from build123d import *

# Parameters (mm, degrees)
SKETCH_1_W          = 1.925
SKETCH_1_H          = 1.2
CUT_EXTRUDE_1_DEPTH = 1
SKETCH_3_W          = 0.8975
SKETCH_3_H          = 0.13363029
EXTRUDE_1_DEPTH     = 0.45
SKETCH_4_W          = 0.13363029
SKETCH_4_H          = 0.8975
EXTRUDE_2_DEPTH     = 0.45
SKETCH_5_W          = 0.8975
SKETCH_5_H          = 0.13363029
EXTRUDE_3_DEPTH     = 0.45
SKETCH_6_W          = 0.13363029
SKETCH_6_H          = 0.8975
EXTRUDE_4_DEPTH     = 0.45
SKETCH_7_R          = 1
EXTRUDE_5_DEPTH     = 6
DRAFT_1_ANGLE       = 30.706601503
DRAFT_2_ANGLE       = 30.706601503
DRAFT_3_ANGLE       = 30.706601503
DRAFT_4_ANGLE       = 30.706601503
FILLET_1_R          = 0.031496063
FILLET_2_R          = 0.45


with BuildPart() as part:
    # 草图1 → 旋转1 (revolve)
    with BuildSketch(Plane.XZ, mode=Mode.PRIVATE) as revolve_1_sk:
        with Locations((0.9625, 0.6)):
            Rectangle(SKETCH_1_W, SKETCH_1_H)
    revolve(revolve_1_sk.sketch.rotate(Axis((0, 0, 1.2), (0, 0, -1)), 270), axis=Axis((0, 0, 1.2), (0, 0, -1)))

    # 草图2 → 切除-拉伸1 (cut)
    with BuildSketch(Plane.XY.offset(1.2)):
        Polygon((0.225, 1.3475), (-0.225, 1.3475), (-0.225, 0.225), (-1.3475, 0.225), (-1.3475, -0.225), (-0.225, -0.225), (-0.225, -1.3475), (0.225, -1.3475), (0.225, -0.225), (1.3475, -0.225), (1.3475, 0.225), (0.225, 0.225), align=None)
    extrude(amount=-CUT_EXTRUDE_1_DEPTH, mode=Mode.SUBTRACT)

    # 草图3 → 凸台-拉伸1 (add)
    with BuildSketch(Plane.XZ.offset(-0.225)):
        with Locations((-0.89875, 0.266815145)):
            Rectangle(SKETCH_3_W, SKETCH_3_H)
    extrude(amount=EXTRUDE_1_DEPTH)

    # 草图4 → 凸台-拉伸2 (add)
    with BuildSketch(Plane(origin=(-0.225, 0, 0), x_dir=(0, 0, -1), z_dir=(1, 0, 0))):
        with Locations((-0.266815145, 0.89875)):
            Rectangle(SKETCH_4_W, SKETCH_4_H)
    extrude(amount=EXTRUDE_2_DEPTH)

    # 草图5 → 凸台-拉伸3 (add)
    with BuildSketch(Plane.XZ.offset(-0.225)):
        with Locations((0.89875, 0.266815145)):
            Rectangle(SKETCH_5_W, SKETCH_5_H)
    extrude(amount=EXTRUDE_3_DEPTH)

    # 草图6 → 凸台-拉伸4 (add)
    with BuildSketch(Plane(origin=(-0.225, 0, 0), x_dir=(0, 0, -1), z_dir=(1, 0, 0))):
        with Locations((-0.266815145, -0.89875)):
            Rectangle(SKETCH_6_W, SKETCH_6_H)
    extrude(amount=EXTRUDE_4_DEPTH)

    # 草图7 → 凸台-拉伸5 (add)
    with BuildSketch(Plane(origin=(0, 0, 0), x_dir=(-1, 0, 0), z_dir=(0, 0, -1))):
        with Locations(Location((0, 0, 0), (0, 0, 90))):
            Circle(SKETCH_7_R)
    extrude(amount=EXTRUDE_5_DEPTH)

    # 拔模1
    draft_1_faces = [part.faces().sort_by_distance(p)[0] for p in [
        (0, 0.89875, 0.33363029),
    ]]
    draft(draft_1_faces, Plane(origin=(0.225, 0.45, 0.2), x_dir=(0, 0, -1), z_dir=(0, -1, 0)), DRAFT_1_ANGLE)

    # 拔模2
    draft_2_faces = [part.faces().sort_by_distance(p)[0] for p in [
        (0.89875, 0, 0.33363029),
    ]]
    draft(draft_2_faces, Plane(origin=(0.45, -0.225, 0.2), x_dir=(0, 0, -1), z_dir=(-1, 0, 0)), DRAFT_2_ANGLE)

    # 拔模3
    draft_3_faces = [part.faces().sort_by_distance(p)[0] for p in [
        (0, -0.89875, 0.33363029),
    ]]
    draft(draft_3_faces, Plane(origin=(0.225, -0.45, 0.33363029), x_dir=(0, 0, 1), z_dir=(0, 1, 0)), DRAFT_3_ANGLE)

    # 拔模4
    draft_4_faces = [part.faces().sort_by_distance(p)[0] for p in [
        (-0.89875, 0, 0.33363029),
    ]]
    draft(draft_4_faces, Plane(origin=(-0.45, -0.225, 0.33363029), x_dir=(0, 0, 1), z_dir=(1, 0, 0)), DRAFT_4_ANGLE)

    # 圆角1
    fillet_1_edges = [part.edges().sort_by_distance(p)[0] for p in [
        (0, -1.925, 1.2),
    ]]
    fillet(fillet_1_edges, radius=FILLET_1_R)

    # 圆角2
    # the kernel refuses this fillet: 0.45 mm, written as the material it takes off along each edge
    with BuildSketch(Plane(origin=(0.225, 0.225, 2.325), x_dir=(0, 1, 0), z_dir=(0, 0, -1))) as fillet_2_piece_1_section:
        with BuildLine():
            CenterArc((FILLET_2_R, FILLET_2_R), FILLET_2_R, 180, 90)
            Line((0, FILLET_2_R), (0, 0))
            Line((0, 0), (FILLET_2_R, 0))
        make_face()
    fillet_2_piece_1 = extrude(amount=3.25, mode=Mode.PRIVATE)
    fillet_2_piece_1 = split(fillet_2_piece_1, bisect_by=Plane(origin=(0.243098692, 0.68726219, 0.474543246), z_dir=(0, -0.5106419849565733, 0.8597934421706244)), keep=Keep.TOP, mode=Mode.PRIVATE)
    fillet_2_piece_1 = split(fillet_2_piece_1, bisect_by=Plane(origin=(0.45, 0.504131357, 0.782889786), z_dir=(-1, 0, 0)), keep=Keep.TOP, mode=Mode.PRIVATE)
    add(fillet_2_piece_1, mode=Mode.SUBTRACT)
    with BuildSketch(Plane(origin=(0.225, 0.225, 2.325), x_dir=(0, 1, 0), z_dir=(0, 0, -1))) as fillet_2_piece_2_section:
        with BuildLine():
            CenterArc((FILLET_2_R, FILLET_2_R), FILLET_2_R, 180, 90)
            Line((0, FILLET_2_R), (0, 0))
            Line((0, 0), (FILLET_2_R, 0))
        make_face()
    fillet_2_piece_2 = extrude(amount=3.25, mode=Mode.PRIVATE)
    fillet_2_piece_2 = split(fillet_2_piece_2, bisect_by=Plane(origin=(0.504131356, 0.45, 0.782889786), z_dir=(0, -1, 0)), keep=Keep.TOP, mode=Mode.PRIVATE)
    fillet_2_piece_2 = split(fillet_2_piece_2, bisect_by=Plane(origin=(0.68726219, 0.243098692, 0.474543246), z_dir=(-0.5106419849565748, 0, 0.8597934421706236)), keep=Keep.TOP, mode=Mode.PRIVATE)
    add(fillet_2_piece_2, mode=Mode.SUBTRACT)
    with BuildSketch(Plane(origin=(0.225, 0.225, 2.325), x_dir=(0, 1, 0), z_dir=(0, 0, -1))) as fillet_2_piece_3_section:
        with BuildLine():
            CenterArc((FILLET_2_R, FILLET_2_R), FILLET_2_R, 180, 90)
            Line((0, FILLET_2_R), (0, 0))
            Line((0, 0), (FILLET_2_R, 0))
        make_face()
    fillet_2_piece_3 = extrude(amount=2.125, mode=Mode.PRIVATE)
    fillet_2_piece_3 = split(fillet_2_piece_3, bisect_by=Plane(origin=(0.325721218, 0.45, 0.219864503), z_dir=(0, -1, 0)), keep=Keep.TOP, mode=Mode.PRIVATE)
    fillet_2_piece_3 = split(fillet_2_piece_3, bisect_by=Plane(origin=(0.45, 0.325721218, 0.219864503), z_dir=(-1, 0, 0)), keep=Keep.TOP, mode=Mode.PRIVATE)
    add(fillet_2_piece_3, mode=Mode.SUBTRACT)
    with BuildSketch(Plane(origin=(0.225, -0.225, 2.325), x_dir=(1, 0, 0), z_dir=(0, 0, -1))) as fillet_2_piece_4_section:
        with BuildLine():
            CenterArc((FILLET_2_R, FILLET_2_R), FILLET_2_R, 180, 90)
            Line((0, FILLET_2_R), (0, 0))
            Line((0, 0), (FILLET_2_R, 0))
        make_face()
    fillet_2_piece_4 = extrude(amount=3.25, mode=Mode.PRIVATE)
    fillet_2_piece_4 = split(fillet_2_piece_4, bisect_by=Plane(origin=(0.68726219, -0.243098692, 0.474543246), z_dir=(-0.5106419849565748, 0, 0.8597934421706236)), keep=Keep.TOP, mode=Mode.PRIVATE)
    fillet_2_piece_4 = split(fillet_2_piece_4, bisect_by=Plane(origin=(0.504131357, -0.45, 0.782889786), z_dir=(0, 1, 0)), keep=Keep.TOP, mode=Mode.PRIVATE)
    add(fillet_2_piece_4, mode=Mode.SUBTRACT)
    with BuildSketch(Plane(origin=(0.225, -0.225, 2.325), x_dir=(1, 0, 0), z_dir=(0, 0, -1))) as fillet_2_piece_5_section:
        with BuildLine():
            CenterArc((FILLET_2_R, FILLET_2_R), FILLET_2_R, 180, 90)
            Line((0, FILLET_2_R), (0, 0))
            Line((0, 0), (FILLET_2_R, 0))
        make_face()
    fillet_2_piece_5 = extrude(amount=3.25, mode=Mode.PRIVATE)
    fillet_2_piece_5 = split(fillet_2_piece_5, bisect_by=Plane(origin=(0.45, -0.504131356, 0.782889786), z_dir=(-1, 0, 0)), keep=Keep.TOP, mode=Mode.PRIVATE)
    fillet_2_piece_5 = split(fillet_2_piece_5, bisect_by=Plane(origin=(0.243098692, -0.68726219, 0.474543246), z_dir=(0, 0.5106419849565746, 0.8597934421706236)), keep=Keep.TOP, mode=Mode.PRIVATE)
    add(fillet_2_piece_5, mode=Mode.SUBTRACT)
    with BuildSketch(Plane(origin=(0.225, -0.225, 2.325), x_dir=(1, 0, 0), z_dir=(0, 0, -1))) as fillet_2_piece_6_section:
        with BuildLine():
            CenterArc((FILLET_2_R, FILLET_2_R), FILLET_2_R, 180, 90)
            Line((0, FILLET_2_R), (0, 0))
            Line((0, 0), (FILLET_2_R, 0))
        make_face()
    fillet_2_piece_6 = extrude(amount=2.125, mode=Mode.PRIVATE)
    fillet_2_piece_6 = split(fillet_2_piece_6, bisect_by=Plane(origin=(0.45, -0.325721218, 0.219864503), z_dir=(-1, 0, 0)), keep=Keep.TOP, mode=Mode.PRIVATE)
    fillet_2_piece_6 = split(fillet_2_piece_6, bisect_by=Plane(origin=(0.325721218, -0.45, 0.219864503), z_dir=(0, 1, 0)), keep=Keep.TOP, mode=Mode.PRIVATE)
    add(fillet_2_piece_6, mode=Mode.SUBTRACT)
    with BuildSketch(Plane(origin=(-0.225, 0.225, 2.325), x_dir=(-1, 0, 0), z_dir=(0, 0, -1))) as fillet_2_piece_7_section:
        with BuildLine():
            CenterArc((FILLET_2_R, FILLET_2_R), FILLET_2_R, 180, 90)
            Line((0, FILLET_2_R), (0, 0))
            Line((0, 0), (FILLET_2_R, 0))
        make_face()
    fillet_2_piece_7 = extrude(amount=3.25, mode=Mode.PRIVATE)
    fillet_2_piece_7 = split(fillet_2_piece_7, bisect_by=Plane(origin=(-0.504131357, 0.45, 0.782889786), z_dir=(0, -1, 0)), keep=Keep.TOP, mode=Mode.PRIVATE)
    fillet_2_piece_7 = split(fillet_2_piece_7, bisect_by=Plane(origin=(-0.68726219, 0.243098692, 0.474543246), z_dir=(0.5106419849565733, 0, 0.8597934421706244)), keep=Keep.TOP, mode=Mode.PRIVATE)
    add(fillet_2_piece_7, mode=Mode.SUBTRACT)
    with BuildSketch(Plane(origin=(-0.225, 0.225, 2.325), x_dir=(-1, 0, 0), z_dir=(0, 0, -1))) as fillet_2_piece_8_section:
        with BuildLine():
            CenterArc((FILLET_2_R, FILLET_2_R), FILLET_2_R, 180, 90)
            Line((0, FILLET_2_R), (0, 0))
            Line((0, 0), (FILLET_2_R, 0))
        make_face()
    fillet_2_piece_8 = extrude(amount=3.25, mode=Mode.PRIVATE)
    fillet_2_piece_8 = split(fillet_2_piece_8, bisect_by=Plane(origin=(-0.243098692, 0.68726219, 0.474543246), z_dir=(0, -0.5106419849565733, 0.8597934421706244)), keep=Keep.TOP, mode=Mode.PRIVATE)
    fillet_2_piece_8 = split(fillet_2_piece_8, bisect_by=Plane(origin=(-0.45, 0.504131356, 0.782889786), z_dir=(1, 0, 0)), keep=Keep.TOP, mode=Mode.PRIVATE)
    add(fillet_2_piece_8, mode=Mode.SUBTRACT)
    with BuildSketch(Plane(origin=(-0.225, 0.225, 2.325), x_dir=(-1, 0, 0), z_dir=(0, 0, -1))) as fillet_2_piece_9_section:
        with BuildLine():
            CenterArc((FILLET_2_R, FILLET_2_R), FILLET_2_R, 180, 90)
            Line((0, FILLET_2_R), (0, 0))
            Line((0, 0), (FILLET_2_R, 0))
        make_face()
    fillet_2_piece_9 = extrude(amount=2.125, mode=Mode.PRIVATE)
    fillet_2_piece_9 = split(fillet_2_piece_9, bisect_by=Plane(origin=(-0.325721218, 0.45, 0.219864503), z_dir=(0, -1, 0)), keep=Keep.TOP, mode=Mode.PRIVATE)
    fillet_2_piece_9 = split(fillet_2_piece_9, bisect_by=Plane(origin=(-0.45, 0.325721218, 0.219864503), z_dir=(1, 0, 0)), keep=Keep.TOP, mode=Mode.PRIVATE)
    add(fillet_2_piece_9, mode=Mode.SUBTRACT)
    with BuildSketch(Plane(origin=(-0.225, -0.225, 2.325), x_dir=(0, -1, 0), z_dir=(0, 0, -1))) as fillet_2_piece_10_section:
        with BuildLine():
            CenterArc((FILLET_2_R, FILLET_2_R), FILLET_2_R, 180, 90)
            Line((0, FILLET_2_R), (0, 0))
            Line((0, 0), (FILLET_2_R, 0))
        make_face()
    fillet_2_piece_10 = extrude(amount=3.25, mode=Mode.PRIVATE)
    fillet_2_piece_10 = split(fillet_2_piece_10, bisect_by=Plane(origin=(-0.243098692, -0.68726219, 0.474543246), z_dir=(0, 0.5106419849565746, 0.8597934421706236)), keep=Keep.TOP, mode=Mode.PRIVATE)
    fillet_2_piece_10 = split(fillet_2_piece_10, bisect_by=Plane(origin=(-0.45, -0.504131357, 0.782889786), z_dir=(1, 0, 0)), keep=Keep.TOP, mode=Mode.PRIVATE)
    add(fillet_2_piece_10, mode=Mode.SUBTRACT)
    with BuildSketch(Plane(origin=(-0.225, -0.225, 2.325), x_dir=(0, -1, 0), z_dir=(0, 0, -1))) as fillet_2_piece_11_section:
        with BuildLine():
            CenterArc((FILLET_2_R, FILLET_2_R), FILLET_2_R, 180, 90)
            Line((0, FILLET_2_R), (0, 0))
            Line((0, 0), (FILLET_2_R, 0))
        make_face()
    fillet_2_piece_11 = extrude(amount=3.25, mode=Mode.PRIVATE)
    fillet_2_piece_11 = split(fillet_2_piece_11, bisect_by=Plane(origin=(-0.504131356, -0.45, 0.782889786), z_dir=(0, 1, 0)), keep=Keep.TOP, mode=Mode.PRIVATE)
    fillet_2_piece_11 = split(fillet_2_piece_11, bisect_by=Plane(origin=(-0.68726219, -0.243098692, 0.474543246), z_dir=(0.5106419849565733, 0, 0.8597934421706244)), keep=Keep.TOP, mode=Mode.PRIVATE)
    add(fillet_2_piece_11, mode=Mode.SUBTRACT)
    with BuildSketch(Plane(origin=(-0.225, -0.225, 2.325), x_dir=(0, -1, 0), z_dir=(0, 0, -1))) as fillet_2_piece_12_section:
        with BuildLine():
            CenterArc((FILLET_2_R, FILLET_2_R), FILLET_2_R, 180, 90)
            Line((0, FILLET_2_R), (0, 0))
            Line((0, 0), (FILLET_2_R, 0))
        make_face()
    fillet_2_piece_12 = extrude(amount=2.125, mode=Mode.PRIVATE)
    fillet_2_piece_12 = split(fillet_2_piece_12, bisect_by=Plane(origin=(-0.325721218, -0.45, 0.219864503), z_dir=(0, 1, 0)), keep=Keep.TOP, mode=Mode.PRIVATE)
    fillet_2_piece_12 = split(fillet_2_piece_12, bisect_by=Plane(origin=(-0.45, -0.325721218, 0.219864503), z_dir=(1, 0, 0)), keep=Keep.TOP, mode=Mode.PRIVATE)
    add(fillet_2_piece_12, mode=Mode.SUBTRACT)


solid = part.part
CAD build for the part. Positions are in the model's coordinates, mm. A direction names the side the tool comes from. Round coordinates to 2 decimals unless told otherwise and drop trailing zeros. Write each loop counter-clockwise with the first axis right and the second up, starting at its lowest first coordinate (ties: lowest second). Pieces come first, ordered by that corner, then holes.
(1) Drop flat-ended pins along their axis: P1, Ø0.5, axis at y = 1, z = 1, coming from the +X side; P2, Ø2, axis at y = 0, z = -2, coming from the +X side; P3, Ø0.7, axis at x = -1, z = 1, coming from the -Y side. Give the stop position or say it passes through.
(2) Slice it at B-B, the plane z = -1.75. Write the cut outline in (x, y), and give its area (3 significant figures).
(3) Probe line 1 along X through (y, z) = (0.05, 0.25); line 2 along Z through (x, y) = (1.4, 0.6); line 3 along X through (y, z) = (-0.85, 0.75) (3 decimals). List the from-to ranges inside material, lowest first.
(4) 3-axis set-ups, long thin cutter, end or side, ignore diameter. For faces 1 (the face through (-1, -1, 0)), 2 (the face through (-0.4, -0.8, 1.2)): which of +Z, -Z, +X, -X, +Y, -Y reach the whole face in a straight line?
(5) Mould opens along X. For faces 3 (the face through (0, 0, 0.2)), 4 (the face through (0, 0, -6)), 5 (the face through (-1, 0, -3)) say: pulls with the +X half, pulls with the -X half, needs draft (parallel to the pull), parting line crosses it, or undercut.
From the geometry:
1. P1: stops at x = 1.77
1. P2: stops at x = 1
1. P3: stops at y = -1.81
2. outline: circle Ø2 at (0, 0)
2. area: 3.14 mm2
3. line 1: x = -1.92 to -0.45, 0.45 to 1.92
3. line 2: z = 0 to 1.2
3. line 3: x = -1.727 to -0.225, 0.225 to 1.727
4. face 1: -Z
4. face 2: +Z, +X, -X, +Y, -Y
5. face 3: undercut
5. face 4: needs draft
5. face 5: parting line crosses it
